```python
from build123d import *

# Parameters (mm, degrees)
F4_W      = 85.725
F4_H      = 47.625
F5_DEPTH  = 3.175
F6_R      = 17.4625
F7_DEPTH  = 30.1625
F8_R      = 17.4625
F9_DEPTH  = 33.3375
F14_SIZE  = 3.175
F15_R     = 4.7625
F16_DEPTH = 7.9375
F17_R     = 2.778125
F18_DEPTH = 25.4


with BuildPart() as f5:
    # F4 (on Front) → F5 (new body, through all)
    with BuildSketch(Plane.XZ):
        Rectangle(F4_W, F4_H)
    extrude(amount=-F5_DEPTH)

    # F6 (on Front) → F7 (join, through all)
    with BuildSketch(Plane.XZ):
        with Locations((19.05, 0)):
            Circle(F6_R)
        with Locations((-19.05, 0)):
            Circle(F6_R)
    extrude(amount=F7_DEPTH)

    # F8 (on Front) → F9 (join, through all)
    with BuildSketch(Plane.XZ):
        with Locations((19.05, 0)):
            Circle(F8_R)
        with Locations((-19.05, 0)):
            Circle(F8_R)
    extrude(amount=-F9_DEPTH)

    # F10 (on plane+point) → F12 (revolve, cut)
    with BuildSketch(Plane.YZ.offset(-19.05)):
        Polygon((0, 14.554762), (-37.202075, 15.204126), (-37.202075, 0), (35.393614, 0), (35.393614, 15.11714), (3.175, 14.554762), (3.175, 11.1125), (0, 11.1125), align=None)
    revolve(axis=Axis((-19.05, -0.90423, 0), (0, 1, 0)), mode=Mode.SUBTRACT)

    # F11 (on plane+point) → F13 (revolve, cut)
    with BuildSketch(Plane.YZ.offset(19.05)):
        Polygon((0, 14.554762), (-37.202075, 15.204126), (-37.202075, 0), (35.393614, 0), (35.393614, 15.11714), (3.175, 14.554762), (3.175, 11.1125), (0, 11.1125), align=None)
    revolve(axis=Axis((19.05, -0.90423, 0), (0, 1, 0)), mode=Mode.SUBTRACT)

    # F14
    f14_edges = [f5.edges().sort_by_distance(p)[0] for p in [
        (-42.8625, 1.5875, 23.8125),
        (42.8625, 1.5875, 23.8125),
        (42.8625, 1.5875, -23.8125),
        (-42.8625, 1.5875, -23.8125),
    ]]
    chamfer(f14_edges, length=F14_SIZE)

    # F15 (on Front) → F16 (join)
    with BuildSketch(Plane.XZ):
        with Locations((36.5125, 17.4625)):
            Circle(F15_R)
        with Locations((-36.5125, 17.4625)):
            Circle(F15_R)
        with Locations((-36.5125, -17.4625)):
            Circle(F15_R)
        with Locations((36.5125, -17.4625)):
            Circle(F15_R)
    extrude(amount=-F16_DEPTH)

    # F17 (on Front) → F18 (cut)
    with BuildSketch(Plane.XZ):
        with Locations((-36.5125, 17.4625)):
            Circle(F17_R)
        with Locations((36.5125, 17.4625)):
            Circle(F17_R)
        with Locations((-36.5125, -17.4625)):
            Circle(F17_R)
        with Locations((36.5125, -17.4625)):
            Circle(F17_R)
    extrude(amount=-F18_DEPTH, mode=Mode.SUBTRACT)


solid = f5.part
```
Input: part model. Units: mm. Frame: model coordinates. A direction names the side the tool comes from. Give positions to 0.01 mm unless a question says otherwise; leave off trailing zeros. Order: outer loops, then holes, each group sorted by start corner. A loop starts at its lowest first (then second) coordinate and runs counter-clockwise, first axis right, second up. Notation, with made-up numbers: M 86.25,-21 L 135.25,-21 A19 ccw 135.25,-5 Z; hole C -39.75,46 d5. An arc over 180 degrees is marked long. Return JSON: item names as keys, results as strings.
Item 1: First-contact query: P1, Ø5, axis at x = -22, z = 10.5, coming from the +Y side (3 decimals); P2, Ø3, axis at x = -38, z = 18.5, coming from the +Y side; P3, Ø1, axis at x = -11.5, z = -4.5, coming from the -Y side; P4, Ø3, axis at y = 7.5, z = 5, coming from the -X side. Flat tips, straight axial feed; report the tip coordinate or a pass-through.
Solutions:
{"P1": "y = 3.175", "P2": "y = 7.94", "P3": "through", "P4": "x = -36.16"}
Item 2: Cut plane A-A (y = 4.5). State how many separate pieces and enclosed holes the cut face has, then the cut area to 3 significant figures.
Solutions:
{"separate pieces": "6", "enclosed holes": "6", "area": "769 mm^2"}
Item 3: Cut plane C-C (x = 37.5). Return loops of the section in (y, z) (1 decimal).
Solutions:
{"outline": "M 0,-23.8 L 3.2,-23.8 L 3.2,-22.1 L 7.9,-22.1 L 7.9,-20.1 L 0,-20.1 Z; M 0,-14.9 L 7.9,-14.9 L 7.9,-12.8 L 3.2,-12.8 L 3.2,12.8 L 7.9,12.8 L 7.9,14.9 L 0,14.9 Z; M 0,20.1 L 7.9,20.1 L 7.9,22.1 L 3.2,22.1 L 3.2,23.8 L 0,23.8 Z"}
Item 4: Ray query, probe 1 along X at (y, z) = (-24, 12.5); probe 2 along X at (y, z) = (-21, -4); probe 3 along X at (y, z) = (7, 16). Return the intervals inside material, ascending.
Solutions:
{"probe 1": "-31.24 to -27.29, -10.81 to -6.86, 6.86 to 10.81, 27.29 to 31.24", "probe 2": "-36.05 to -33.43, -4.67 to -2.05, 2.05 to 4.67, 33.43 to 36.05", "probe 3": "-41.04 to -38.87, -34.15 to -31.98, -26.05 to -12.05, 12.05 to 26.05, 31.98 to 34.15, 38.87 to 41.04"}
Item 5: Pull-direction query (Z, two-part tool) for faces 6 (the flat face through (-24.3, -30.162, 14.3)), 7 (the flat face through (-1, 2, -23.812)), 8 (the flat face through (-30, 0, 3)); classes: +Z half, -Z half, draft (parallel to the pull), parting line (faces both ways), or undercut.
Solutions:
{"face 6": "draft", "face 7": "-Z half", "face 8": "undercut"}
Item 6: Access query for faces 1 (the conical face through (4.58, -15.29, -3.21)), 2 (the flat face through (-34, 7.938, 15)), 3 (the flat face through (-1, 3.175, 0)), 4 (the flat face through (-34, 7.938, -20)), 5 (the flat face through (39, 7.938, 15)). Directions: +Z, -Z, +X, -X, +Y, -Y. A direction counts if a zero-diameter tool reaches every point of the face in a straight line with its end or side. Return the directions, or none.
Solutions:
{"face 1": "-Y", "face 2": "+Z, -X, +Y", "face 3": "+Y", "face 4": "-Z, -X, +Y", "face 5": "+Z, +X, +Y"}
Item 7: Cut plane B-B (z = -19). Return loops of the section in (x, y) (1 decimal).
Solutions:
{"outline": "M -42.9,0 L -38.8,0 L -38.8,7.9 L -41,7.9 L -41,3.2 L -42.9,3.2 Z; M -34.2,0 L 34.2,0 L 34.2,7.9 L 32,7.9 L 32,3.2 L -32,3.2 L -32,7.9 L -34.2,7.9 Z; M 38.8,0 L 42.9,0 L 42.9,3.2 L 41,3.2 L 41,7.9 L 38.8,7.9 Z"}
